```python
from build123d import *

# Parameters (mm, degrees)
SKETCH_1_W          = 20
SKETCH_1_H          = 100
EXTRUDE_1_DEPTH     = 4
SKETCH_2_R          = 2.5
CUT_EXTRUDE_1_DEPTH = 103.058806577
SKETCH_3_W          = 20
SKETCH_3_H          = 10
CUT_EXTRUDE_2_DEPTH = 2
CUT_EXTRUDE_3_DEPTH = 103.058806577


with BuildPart() as part:
    # 草图1 → 凸台-拉伸1 (new body)
    with BuildSketch(Plane.XY):
        with Locations((10, -50)):
            Rectangle(SKETCH_1_W, SKETCH_1_H)
    extrude(amount=EXTRUDE_1_DEPTH)

    # 草图2 → 切除-拉伸1 (cut, through all)
    with BuildSketch(Plane.XY.offset(4)):
        with Locations((5, -5)):
            Circle(SKETCH_2_R)
        with Locations((15, -5)):
            Circle(SKETCH_2_R)
    extrude(amount=-CUT_EXTRUDE_1_DEPTH, mode=Mode.SUBTRACT)

    # 草图3 → 切除-拉伸2 (cut)
    with BuildSketch(Plane(origin=(0, 0, 0), x_dir=(-1, 0, 0), z_dir=(0, 0, -1))):
        with Locations((-10, -5)):
            Rectangle(SKETCH_3_W, SKETCH_3_H)
    extrude(amount=-CUT_EXTRUDE_2_DEPTH, mode=Mode.SUBTRACT)

    # 草图4 → 切除-拉伸3 (cut, through all)
    with BuildSketch(Plane.XY.offset(4)):
        Polygon((0, -90), (0, -100), (8, -100), align=None)
        Polygon((20, -100), (12, -100), (20, -90), align=None)
    extrude(amount=-CUT_EXTRUDE_3_DEPTH, mode=Mode.SUBTRACT)


solid = part.part
```
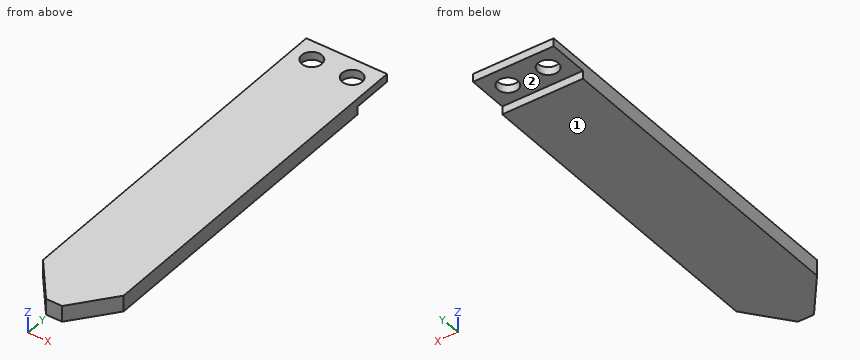
Check sheet for the modelled part. Datum: model origin and axes. Units: mm. Face numbers are marked on the shaded views. A direction names the side the tool comes from. Coordinates: 2 decimals unless noted, no trailing zeros. Write each loop counter-clockwise with the first axis right and the second up, starting at its lowest first coordinate (ties: lowest second). Pieces come first, ordered by that corner, then holes. Notation, with made-up numbers: (59, 19) -> (86, 19) arc R31 ccw to (86, 52) -> close; hole circle Ø6 at (29, -3). An arc over 180 degrees is marked (long way). Use a Markdown table: item, result.
1. Sectioned sample at D-D (x = 10). Enter the section's corners in (y, z), plus the area to 3 significant figures.
Reported:
| item | result |
|---|---|
| outline | (-100, 0) -> (-10, 0) -> (-10, 2) -> (0, 2) -> (0, 4) -> (-100, 4) -> close |
| area | 380 mm2 |
2. Go/stop test with a flat-tipped pin: pin 1 Ø6 at (x, y) = (15, -5) entering from -Z. Record where the tip stops, or that it passes through.
Reported:
| item | result |
|---|---|
| pin 1 | stops at z = 2 |
3. Sectioned sample at A-A (y = -5). Enter the section's corners in (x, z).
Reported:
| item | result |
|---|---|
| outline | (0, 2) -> (2.5, 2) -> (2.5, 4) -> (0, 4) -> close; (7.5, 2) -> (12.5, 2) -> (12.5, 4) -> (7.5, 4) -> close; (17.5, 2) -> (20, 2) -> (20, 4) -> (17.5, 4) -> close |
4. Scan lines: line 1 along Z through (x, y) = (12.25, -8.5); line 2 along Y through (x, z) = (5, 3.4); line 3 along Y through (x, z) = (15.75, 2.55). Record each from-to range of solid material in increasing order.
Reported:
| item | result |
|---|---|
| line 1 | z = 2 to 4 |
| line 2 | y = -96.25 to -7.5, -2.5 to 0 |
| line 3 | y = -95.31 to -7.38, -2.62 to 0 |
5. Sectioned sample at B-B (x = 5). Enter the section's corners in (y, z), plus the area to 3 significant figures.
Reported:
| item | result |
|---|---|
| outline | (-96.25, 0) -> (-10, 0) -> (-10, 2) -> (-7.5, 2) -> (-7.5, 4) -> (-96.25, 4) -> close; (-2.5, 2) -> (0, 2) -> (0, 4) -> (-2.5, 4) -> close |
| area | 355 mm2 |
6. Sectioned sample at C-C (z = 3.25). Enter the section's corners in (x, y), plus the area to 3 significant figures.
Reported:
| item | result |
|---|---|
| outline | (0, -90) -> (8, -100) -> (12, -100) -> (20, -90) -> (20, 0) -> (0, 0) -> close; hole circle Ø5 at (5, -5); hole circle Ø5 at (15, -5) |
| area | 1,880 mm2 |
7. Tool access check on the marked faces 1 and 2. Record the directions out of +Z, -Z, +X, -X, +Y, -Y that give a thin tool (end or side, any length) a straight path to the whole face; none if there is none.
Reported:
| item | result |
|---|---|
| face 1 | -Z, +X, -X, +Y, -Y |
| face 2 | -Z, +X, -X, +Y |
